Read the model definition and answer for the solid it produces. Units are mm, in the model's axes. Face numbers are marked on the shaded views. A direction names the side the tool comes from. Coordinates: 2 decimals unless noted, no trailing zeros. Write each loop counter-clockwise with the first axis right and the second up, starting at its lowest first coordinate (ties: lowest second). Pieces come first, ordered by that corner, then holes.
Item 1: Each of these flat-tipped pins is pushed along its axis until it touches: P1, Ø14.5, axis at y = -33.5, z = 9, coming from the +X side; P2, Ø10, axis at x = 21.5, z = 23, coming from the -Y side. Where does it stop, or does it pass through?
Item 2: A tool of negligible diameter and unlimited length cuts with its end or side. For the marked faces 5 and 6, from which of +Z, -Z, +X, -X, +Y, -Y can it reach the whole face along a straight path? Write none if from no direction.
Item 3: Section C-C (x = 25) is taken. Give the vertices of the cut face in (y, z), then the cut area to 3 significant figures.
Item 4: Determine the mould class of the marked faces 1, 2, 3 and 4 for opening direction X: released by +X, released by -X, zero draft, split by the parting line, or undercut.
Item 5: Section B-B (z = 25) is taken. Give the vertices of the cut face in (x, y).
Item 6: Straight lines are drawn through the part: probe 1 along Z at (x, y) = (25, -7); probe 2 along Y at (x, z) = (32, 20.75); probe 3 along Y at (x, z) = (9.25, 24). For each, find the intervals that lie inside material, in ascending order.
Item 7: Section A-A (y = -43) is taken. Give the vertices of the cut face in (x, z).
Item 8: Section D-D (x = 31.5) is taken. Give the vertices of the cut face in (y, z), then the cut area to 3 significant figures.
from build123d import *

# Parameters (mm, degrees)
SKETCH1_R           = 4
BOSS_EXTRUDE1_DEPTH = 32
SKETCH2_R           = 4
CUT_EXTRUDE1_DEPTH  = 75.813100457
CUT_EXTRUDE2_DEPTH  = 61.241181927
CHAMFER1_SIZE       = 5
CHAMFER1_SIZE2      = 3
CHAMFER2_SIZE       = 3
CHAMFER2_SIZE2      = 5


with BuildPart() as part:
    # Sketch1 → Boss-Extrude1 (new body)
    with BuildSketch(Plane.XY):
        Polygon((42, 0), (42, -24), (13, -24), (13, -53), (0, -53), (0, 0), align=None)
        with Locations((32, -12)):
            Circle(SKETCH1_R, mode=Mode.SUBTRACT)
    extrude(amount=BOSS_EXTRUDE1_DEPTH)

    # Sketch2 → Cut-Extrude1 (cut, through all)
    with BuildSketch(Plane.ZY):
        with Locations((8, -43)):
            Circle(SKETCH2_R)
        with Locations((24, -43)):
            Circle(SKETCH2_R)
    extrude(amount=-CUT_EXTRUDE1_DEPTH, mode=Mode.SUBTRACT)

    # Sketch3 → Cut-Extrude2 (cut, through all)
    with BuildSketch(Plane.XZ.offset(24)):
        with BuildLine():
            Line((32.348469228, 17.5), (42, 17.5))
            Line((42, 17.5), (42, 14.5))
            Line((42, 14.5), (32.348469228, 14.5))
            ThreePointArc((32.348469228, 14.5), (17.5, 16), (32.348469228, 17.5))
        make_face()
    extrude(amount=-CUT_EXTRUDE2_DEPTH, mode=Mode.SUBTRACT)

    # Chamfer1
    chamfer1_edges = [part.edges().sort_by_distance(p)[0] for p in [
        (42, -12, 32),
    ]]
    chamfer1_side = [part.faces().sort_by_distance(p)[0] for p in [
        (16.490174092, -19.485009093, 32),
    ]]
    chamfer(chamfer1_edges, length=CHAMFER1_SIZE, length2=CHAMFER1_SIZE2, reference=chamfer1_side[0])

    # Chamfer2
    chamfer2_edges = [part.edges().sort_by_distance(p)[0] for p in [
        (42, -12, 0),
    ]]
    chamfer2_side = [part.faces().sort_by_distance(p)[0] for p in [
        (42, -12, 7.25),
    ]]
    chamfer(chamfer2_edges, length=CHAMFER2_SIZE, length2=CHAMFER2_SIZE2, reference=chamfer2_side[0])


solid = part.part
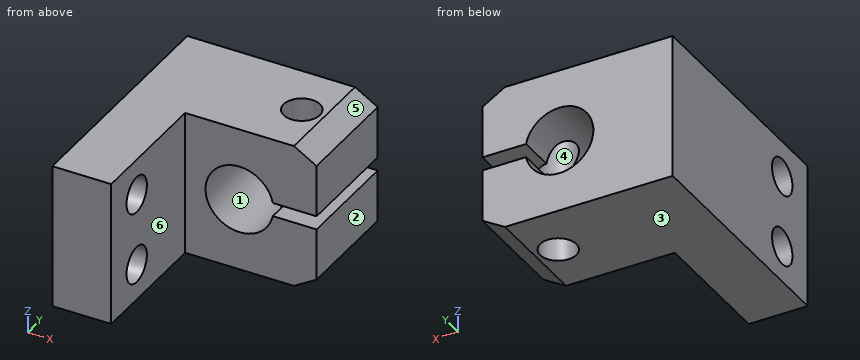
Established:
1. P1: stops at x = 13
1. P2: stops at y = -24
2. face 5: +Z, +X, +Y, -Y
2. face 6: +Z, -Z, +X, -Y
3. outline: (-24, 0) - (0, 0) - (0, 8.5) - (-24, 8.5) - close; (-24, 23.5) - (0, 23.5) - (0, 32) - (-24, 32) - close
3. area: 408 mm2
4. face 1: undercut
4. face 2: released by +X
4. face 3: zero draft
4. face 4: undercut
5. outline: (0, -53) - (13, -53) - (13, -46.87) - (0, -46.87) - close; (0, -39.13) - (13, -39.13) - (13, -24) - (42, -24) - (42, 0) - (0, 0) - close; hole circle Ø8 at (32, -12)
6. probe 1: z = 0 to 8.5, 23.5 to 32
6. probe 2: y = -24 to -16, -8 to 0
6. probe 3: y = -53 to -47, -39 to 0
7. outline: (0, 0) - (13, 0) - (13, 4) - (0, 4) - close; (0, 12) - (13, 12) - (13, 20) - (0, 20) - close; (0, 28) - (13, 28) - (13, 32) - (0, 32) - close
8. outline: (-24, 0) - (-15.97, 0) - (-15.97, 12.26) - (-24, 12.26) - close; (-24, 19.74) - (-15.97, 19.74) - (-15.97, 32) - (-24, 32) - close; (-8.03, 0) - (0, 0) - (0, 12.26) - (-8.03, 12.26) - close; (-8.03, 19.74) - (0, 19.74) - (0, 32) - (-8.03, 32) - close
8. area: 394 mm2
